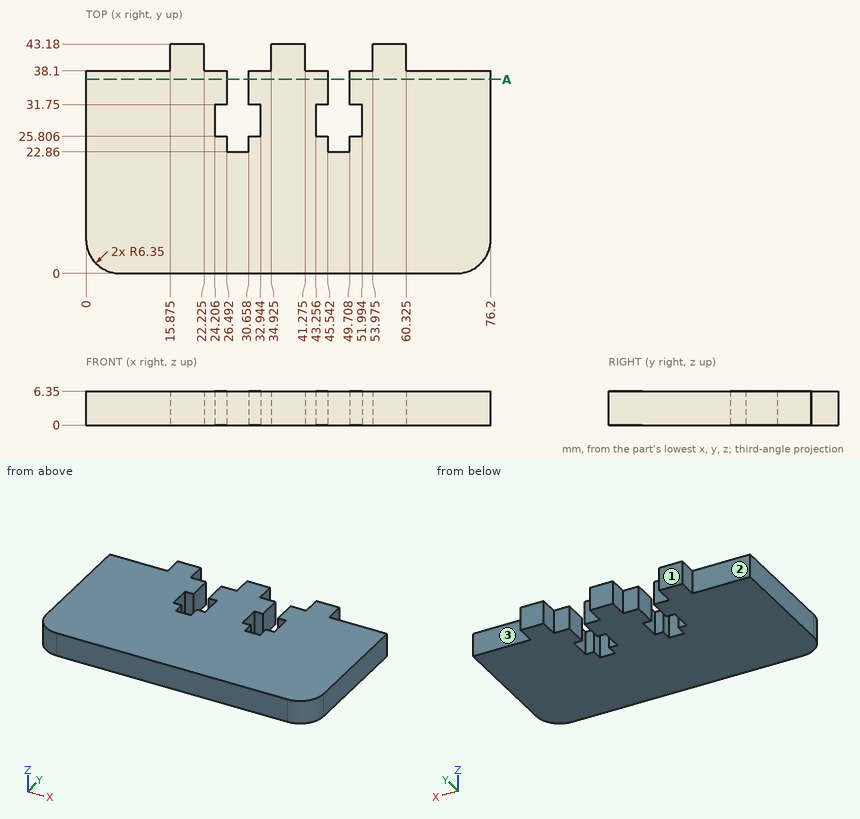
For this review, use the dimensioned drawing (mm, ordinates from the lowest corner) and the shaded views. A direction names the side the tool comes from. Round coordinates to 2 decimals unless told otherwise and drop trailing zeros. Order: outer loops, then holes, each group sorted by start corner. A loop starts at its lowest first (then second) coordinate and runs counter-clockwise, first axis right, second up. Notation, with made-up numbers: M -28.5,35 L -19.5,35 A18 cw -19.5,45 Z; hole C -6.75,22.5 d4. An arc over 180 degrees is marked long. Write each question's results on one line, items separated by ' | '. Start each with the question number.
1. Clearance check with flat-ended pins moving along their axes: pin 1 Ø1.1 at (x, z) = (25, 1.5) entering from -Y; pin 2 Ø2 at (x, z) = (47.5, 3.5) entering from +Y; pin 3 Ø3.5 at (x, z) = (52, 3.5) entering from +Y. State where each tip first meets the part, or that it passes through.
2. Add section A-A (y = 36.5). State the section outline as (x, z) points, then the cut area to 3 significant figures.
3. Tool access review of the marked faces 1, 2 and 3: name each direction out of +Z, -Z, +X, -X, +Y, -Y from which nothing blocks a thin tool from reaching the whole face with its end or side.
4. To check wall thickness, follow L1, parallel to X at y = 32.5, z = 3.5; L2, parallel to X at y = 28, z = 2; L3, parallel to Y at x = 50.5, z = 3.75. State the ranges of each line that lie inside material, in increasing order. Write a range as [from, to].
Output values:
1) pin 1: y = 0 | pin 2: y = 22.86 | pin 3: y = 38.1
2) outline: M 0,0 L 26.49,0 L 26.49,6.35 L 0,6.35 Z; M 30.66,0 L 45.54,0 L 45.54,6.35 L 30.66,6.35 Z; M 49.71,0 L 76.2,0 L 76.2,6.35 L 49.71,6.35 Z | area: 431 mm^2
3) face 1: +Z, -Z, +X, -X, +Y | face 2: +Z, -Z, -X, +Y | face 3: +Z, -Z, +X, +Y
4) L1: [0, 26.49], [30.66, 45.54], [49.71, 76.2] | L2: [0, 24.21], [32.94, 43.26], [51.99, 76.2] | L3: [0, 25.81], [31.75, 38.1]
